from build123d import *

# Parameters (mm, degrees)
SKETCH1_W           = 31.8
SKETCH1_H           = 7.8
BOSS_EXTRUDE1_DEPTH = 4.9
SKETCH2_R           = 2.4
BOSS_EXTRUDE2_DEPTH = 1.8
SKETCH3_W           = 28.6
SKETCH3_H           = 4.6
CUT_EXTRUDE1_DEPTH  = 8
SKETCH6_R           = 1.5
BOSS_EXTRUDE3_DEPTH = 8


with BuildPart() as part:
    # Sketch1 → Boss-Extrude1 (new body, symmetric)
    with BuildSketch(Plane(origin=(0, 0, 0), x_dir=(1, 0, 0), z_dir=(0, 1, 0))):
        Rectangle(SKETCH1_W, SKETCH1_H)
    extrude(amount=BOSS_EXTRUDE1_DEPTH, both=True)

    # Sketch2 → Boss-Extrude2 (add)
    with BuildSketch(Plane(origin=(15.9, 4.9, -3.9), x_dir=(1, 0, 0), z_dir=(0, -1, 0))):
        with Locations((-27.804807902, 3.9)):
            Circle(SKETCH2_R)
        with Locations((-19.804807902, 3.9)):
            Circle(SKETCH2_R)
        with Locations((-11.804807902, 3.9)):
            Circle(SKETCH2_R)
        with Locations((-3.804807902, 3.9)):
            Circle(SKETCH2_R)
    extrude(amount=-BOSS_EXTRUDE2_DEPTH)

    # Sketch3 → Cut-Extrude1 (cut)
    with BuildSketch(Plane.XZ.offset(4.9)):
        Rectangle(SKETCH3_W, SKETCH3_H)
    extrude(amount=-CUT_EXTRUDE1_DEPTH, mode=Mode.SUBTRACT)

    # Sketch6 → Boss-Extrude3 (add)
    with BuildSketch(Plane(origin=(15.9, 3.3, -3.9), x_dir=(-1, 0, 0), z_dir=(0, -1, 0))):
        with Locations((7.95, -3.9)):
            Circle(SKETCH6_R)
        with Locations((15.9, -3.9)):
            Circle(SKETCH6_R)
        with Locations((23.85, -3.9)):
            Circle(SKETCH6_R)
    extrude(amount=BOSS_EXTRUDE3_DEPTH)


solid = part.part
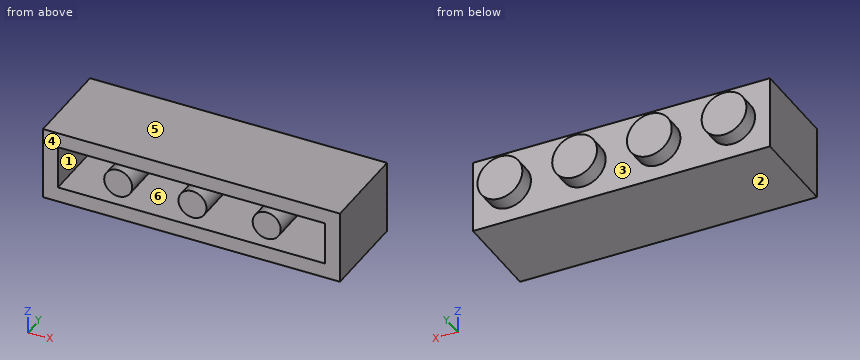
The listing builds one solid part. Answer for the finished solid, in the listing's coordinates (mm). Face numbers are marked on the shaded views. A direction names the side the tool comes from. Round coordinates to 2 decimals unless told otherwise and drop trailing zeros. Order: outer loops, then holes, each group sorted by start corner. A loop starts at its lowest first (then second) coordinate and runs counter-clockwise, first axis right, second up. Notation, with made-up numbers: M 47,30 L 68,30 A34 cw 68,63 Z; hole C -33.75,-36.5 d6. An arc over 180 degrees is marked long. Answer in a Markdown table with one row per item. Add a question column.
1) Which of the six approach directions +Z, -Z, +X, -X, +Y, -Y give full straight-line access (tool end or side, diameter ignored) to the marked faces 1, 2 and 3?
2) The part is cut by section A-A on x = 7.95. Determine the outline of the cut face in (y, z).
3) Consider line 1 along X through (y, z) = (-2.5, -1.25); line 2 along Z through (x, y) = (8.5, 2.5); line 3 along X through (y, z) = (-3.5, -1). Determine where each line is inside the solid, lowest interval first. Write a range as from..to.
4) The part is cut by section B-B on y = 5.5. Determine the outline of the cut face in (x, z), plus the area to 3 significant figures.
5) The part is cut by section C-C on z = -2. Determine the outline of the cut face in (x, y), plus the area to 3 significant figures.
6) Determine the mould class of the marked faces 4, 5 and 6 for opening direction Z: pulls with the +Z half, pulls with the -Z half, needs draft (parallel to the pull), parting line crosses it, or undercut.
7) Flat-ended cylindrical pins translate along their axes: pin 1 Ø3.5 at (x, z) = (-7.5, -0.5) entering from -Y; pin 2 Ø3.5 at (x, z) = (-3.5, -0.5) entering from -Y; pin 3 Ø2 at (x, z) = (-7.5, 3) entering from +Y. Find the tip coordinate at first contact, or state that the pin passes through.
8) The part is cut by section D-D on x = -12. Determine the outline of the cut face in (y, z).
Findings below:
| question | item | result |
|---|---|---|
| 1 | face 1 | -Y |
| 1 | face 2 | -Z, +X, -X, +Y, -Y |
| 1 | face 3 | +Y |
| 2 | outline | M -4.9,-3.9 L 4.9,-3.9 L 4.9,3.9 L -4.9,3.9 L -4.9,2.3 L 3.1,2.3 L 3.1,1.5 L -4.7,1.5 L -4.7,-1.5 L 3.1,-1.5 L 3.1,-2.3 L -4.9,-2.3 Z |
| 3 | line 1 | x = -15.9..-14.3, -8.78..-7.12, -0.83..0.83, 7.12..8.78, 14.3..15.9 |
| 3 | line 2 | z = -3.9..-2.3, -1.4..1.4, 2.3..3.9 |
| 3 | line 3 | x = -15.9..-14.3, -9.07..-6.83, -1.12..1.12, 6.83..9.07, 14.3..15.9 |
| 4 | outline | C -11.9,0 d4.8; C -3.9,0 d4.8; C 4.1,0 d4.8; C 12.1,0 d4.8 |
| 4 | area | 72.4 mm² |
| 5 | outline | M -15.9,-4.9 L -14.3,-4.9 L -14.3,3.1 L 14.3,3.1 L 14.3,-4.9 L 15.9,-4.9 L 15.9,4.9 L 13.42,4.9 L 13.42,6.7 L 10.77,6.7 L 10.77,4.9 L 5.42,4.9 L 5.42,6.7 L 2.77,6.7 L 2.77,4.9 L -2.58,4.9 L -2.58,6.7 L -5.23,6.7 L -5.23,4.9 L -10.58,4.9 L -10.58,6.7 L -13.23,6.7 L -13.23,4.9 L -15.9,4.9 Z |
| 5 | area | 102 mm² |
| 6 | face 4 | needs draft |
| 6 | face 5 | pulls with the +Z half |
| 6 | face 6 | undercut |
| 7 | pin 1 | stops at y = -4.7 |
| 7 | pin 2 | stops at y = 3.1 |
| 7 | pin 3 | stops at y = 4.9 |
| 8 | outline | M -4.9,-3.9 L 4.9,-3.9 L 4.9,-2.4 L 6.7,-2.4 L 6.7,2.4 L 4.9,2.4 L 4.9,3.9 L -4.9,3.9 L -4.9,2.3 L 3.1,2.3 L 3.1,-2.3 L -4.9,-2.3 Z |
